Input: part model. Units: mm. Frame: model coordinates. A direction names the side the tool comes from. Coordinates: 2 decimals unless noted, no trailing zeros. Loops run counter-clockwise (first coordinate to the right, second up) from the corner with the lowest first, then second, coordinate; pieces in that order, holes last. Notation, with made-up numbers: (3, 60) - (55, 60) arc R17 cw to (55, 89) - close; hole circle Ø6 at (-24, 26.5). An arc over 180 degrees is marked (long way). Use a Markdown table: item, result. Add a question column.
1. Section query A-A on x = 0. Return the cut outline in (y, z).
2. Section query C-C on z = 2.5. Return the cut outline in (x, y), then the cut area to 3 significant figures.
3. Section query D-D on x = 6.5. Return the cut outline in (y, z), then the cut area to 3 significant figures.
4. Access query for faces 1 (the face through (7, 1, -2)), 2 (the face through (18, 0, -2)), 3 (the face through (25.38, 1.48, -2.07)). Directions: +Z, -Z, +X, -X, +Y, -Y. A direction counts if a zero-diameter tool reaches every point of the face in a straight line with its end or side. Return the directions, or none.
5. Section query B-B on y = 0.55. Return the cut outline in (x, z).
6. Draft query along Z for faces 4 (the face through (13.788, 1.479, 5.443)), 5 (the face through (11.5, 1.48, -0.07)), 6 (the face through (24.301, 1.479, -5.928)). Return one class per face: released by +Z, released by -Z, zero draft, split by the parting line, or undercut.
7. Ray query, L1, parallel to Z at x = 0, y = 1.85; L2, parallel to Z at x = 37.5, y = 1.45; L3, parallel to X at y = 1.4, z = -10.25. Return the intervals inside material, ascending. Write a range as [from, to].
8. Contact query for flat-ended pins moving along their axis: P1, Ø1.5, axis at y = 2.5, z = 3.5, coming from the -X side; P2, Ø0.8, axis at x = 6, y = 1.5, coming from the -Z side; P3, Ø1.8, axis at x = 0, z = 0, coming from the -Y side. Output: stop coordinate, or through.
```python
from build123d import *

# Parameters (mm, degrees)
SKETCH1_R           = 1.5
BOSS_EXTRUDE1_DEPTH = 3


with BuildPart() as part:
    # Sketch1 → Boss-Extrude1 (new body)
    with BuildSketch(Plane(origin=(0, 0, 0), x_dir=(1, 0, 0), z_dir=(0, 1, 0))):
        with BuildLine():
            ThreePointArc((5.123475383, 2), (-5.5, 0), (5.123475383, -2))
            Line((5.123475383, -2), (7.876524617, -2))
            ThreePointArc((7.876524617, -2), (13.891801362, -5.42721755), (18.494070457, -0.255322963))
            Line((18.494070457, -0.255322963), (32.471368108, 4.465652792))
            ThreePointArc((32.471368108, 4.465652792), (41.896235049, 9.76), (31.191368108, 8.255322963))
            Line((31.191368108, 8.255322963), (17.214070457, 3.534347208))
            ThreePointArc((17.214070457, 3.534347208), (12.108198638, 5.42721755), (7.876524617, 2))
            Line((7.876524617, 2), (5.123475383, 2))
        make_face()
        Circle(SKETCH1_R, mode=Mode.SUBTRACT)
        with Locations((13, 0)):
            Circle(SKETCH1_R, mode=Mode.SUBTRACT)
        with Locations((36.685438565, 8)):
            Circle(SKETCH1_R, mode=Mode.SUBTRACT)
    extrude(amount=BOSS_EXTRUDE1_DEPTH)


solid = part.part
```
Resolved:
| question | item | result |
|---|---|---|
| 1 | outline | (0, -5.5) - (3, -5.5) - (3, -1.5) - (0, -1.5) - close; (0, 1.5) - (3, 1.5) - (3, 5.5) - (0, 5.5) - close |
| 2 | outline | (-4.9, 0) - (4.9, 0) - (4.9, 3) - (-4.9, 3) - close; (8.1, 0) - (17.9, 0) - (17.9, 3) - (8.1, 3) - close |
| 2 | area | 58.8 mm² |
| 3 | outline | (0, -2) - (3, -2) - (3, 2) - (0, 2) - close |
| 3 | area | 12.0 mm² |
| 4 | face 1 | -Z, +Y, -Y |
| 4 | face 2 | +Z, -Z, +X, -X, -Y |
| 4 | face 3 | +Z, +Y, -Y |
| 5 | outline | (5.12, -2) - (7.88, -2) arc R5.5 ccw to (17.21, -3.53) - (31.19, -8.26) arc R5.5 ccw (long way) to (32.47, -4.47) - (18.49, 0.26) arc R5.5 ccw to (7.88, 2) - (5.12, 2) arc R5.5 ccw (long way) to start; hole circle Ø3 at (0, 0); hole circle Ø3 at (13, 0); hole circle Ø3 at (36.69, -8) |
| 6 | face 4 | released by +Z |
| 6 | face 5 | undercut |
| 6 | face 6 | released by -Z |
| 7 | L1 | [-5.5, -1.5], [1.5, 5.5] |
| 7 | L2 | [-13.44, -9.26], [-6.74, -2.56] |
| 7 | L3 | [31.67, 41.7] |
| 8 | P1 | x = -4.76 |
| 8 | P2 | z = -2 |
| 8 | P3 | through |
